Can you work these out from the model? Positions are in its coordinate system, mm. Coordinates: 2 decimals unless noted, no trailing zeros. Order: outer loops, then holes, each group sorted by start corner. A loop starts at its lowest first (then second) coordinate and runs counter-clockwise, first axis right, second up. Notation, with made-up numbers: (44, 1.5) - (69, 1.5) arc R27 ccw to (69, 22.5) - close; hole circle Ø3 at (-5, -29). An arc over 180 degrees is marked (long way). Return JSON: item names as keys, results as strings. Group by question number.
1) Imagine slicing it at C-C (y = -13.5). Write out the boundary of the cut face in (x, z), and give its area (3 significant figures).
2) If I drill on line 1 along Y through (x, z) = (436.5, 16.25); line 2 along Z through (x, y) = (182, -52); line 3 along Y through (x, z) = (67, 15.5), over which ranges is the centre line in solid material (lowest first)?
3) Imagine slicing it at B-B (z = 12). Give the number of separate pieces and of enclosed holes in the cut face, and give its area (3 significant figures).
4) For pin 1 Ø2 at (x, z) = (128.5, 10.5) entering from +Y; pin 2 Ø1 at (y, z) = (3, 17.5) entering from +X; pin 3 Ø1.5 at (x, z) = (218, 16) entering from +Y, each with a flat end and sliding along its axis, tell me the tip position at first contact or that it passes through.
5) Imagine slicing it at A-A (x = 46). Write out the boundary of the cut face in (y, z), and give its area (3 significant figures).
```python
from build123d import *

# Parameters (mm, degrees)
F0_W     = 505.468076095
F0_H     = 137.6467421651
F1_DEPTH = 7.366
F3_DEPTH = 12.446


# Not quite as in the source:
# - a feature names something its author has since deleted; it is built from what else it names


with BuildPart() as f1:
    # F0 (on Top) → F1 (new body)
    with BuildSketch(Plane.XY):
        with Locations((232.2135167196, 0.7967613637)):
            Rectangle(F0_W, F0_H)
    extrude(amount=F1_DEPTH)

    # F2 (on face) → F3 (join)
    with BuildSketch(Plane.XY.offset(7.366)):
        with BuildLine():
            Line((183.8642209768, 14.1799058765), (183.8642209768, 10.2725932375))
            Line((183.8642209768, 10.2725932375), (181.7528605461, 10.280970484))
            Line((181.7528605461, 10.280970484), (174.2617040873, 10.3483377025))
            Line((174.2617040873, 10.3483377025), (137.7773582935, 10.3483377025))
            Line((137.7773582935, 10.3483377025), (125.377446413, 4.0150946006))
            Line((125.377446413, 4.0150946006), (138.0158215761, -2.1848597098))
            Line((138.0158215761, -2.1848597098), (174.0232408047, -2.1848597098))
            Line((174.0232408047, -2.1848597098), (181.7289143801, -2.1529737648))
            Line((181.7289143801, -2.1529737648), (183.6102157831, -2.1509330043))
            Line((183.6102157831, -2.1509330043), (183.5907548666, -5.8423327282))
            Line((183.5907548666, -5.8423327282), (186.6615414619, -5.8423327282))
            Line((186.6615414619, -5.8423327282), (186.6615414619, -2.0806165412))
            Line((186.6615414619, -2.0806165412), (189.655572176, -2.0806165412))
            Line((189.655572176, -2.0806165412), (189.655572176, -5.8423327282))
            Line((189.655572176, -5.8423327282), (192.6495879889, -5.8423327282))
            Line((192.6495879889, -5.8423327282), (192.6495879889, -2.0806165412))
            Line((192.6495879889, -2.0806165412), (195.8739161491, -2.0806165412))
            Line((195.8739161491, -2.0806165412), (195.8739161491, -5.8423327282))
            Line((195.8739161491, -5.8423327282), (199.0982443094, -5.8423327282))
            Line((199.0982443094, -5.8423327282), (199.0982443094, -2.0806165412))
            Line((199.0982443094, -2.0806165412), (202.4761140347, -2.0806165412))
            Line((202.4761140347, -2.0806165412), (202.4761140347, -5.8423327282))
            Line((202.4761140347, -5.8423327282), (206.2378227711, -5.8423327282))
            Line((206.2378227711, -5.8423327282), (206.2378227711, -2.0806165412))
            Line((206.2378227711, -2.0806165412), (209.6156924963, -2.0806165412))
            Line((209.6156924963, -2.0806165412), (209.6156924963, -5.8423327282))
            Line((209.6156924963, -5.8423327282), (213.1471037865, -5.8423327282))
            Line((213.1471037865, -5.8423327282), (213.1471037865, -2.0806165412))
            Line((213.1471037865, -2.0806165412), (216.1411345005, -2.0806165412))
            Line((216.1411345005, -2.0806165412), (216.1411345005, -5.8423327282))
            Line((216.1411345005, -5.8423327282), (219.1351503134, -5.8423327282))
            Line((219.1351503134, -5.8423327282), (219.1351503134, -2.0806165412))
            Line((219.1351503134, -2.0806165412), (222.3594784737, -2.0806165412))
            Line((222.3594784737, -2.0806165412), (222.3594784737, -5.8423327282))
            Line((222.3594784737, -5.8423327282), (225.5838066339, -5.8423327282))
            Line((225.5838066339, -5.8423327282), (225.5838066339, -2.0806165412))
            Line((225.5838066339, -2.0806165412), (228.9616763592, -2.0806165412))
            Line((228.9616763592, -2.0806165412), (228.9616763592, -5.8423327282))
            Line((228.9616763592, -5.8423327282), (232.7233850956, -5.8423327282))
            Line((232.7233850956, -5.8423327282), (232.7233850956, -2.0806165412))
            Line((232.7233850956, -2.0806165412), (236.1012548208, -2.0806165412))
            Line((236.1012548208, -2.0806165412), (236.1012548208, -5.8423327282))
            Line((236.1012548208, -5.8423327282), (239.886666111, -5.8423327282))
            Line((239.886666111, -5.8423327282), (239.886666111, -2.0361929703))
            Line((239.886666111, -2.0361929703), (308.7113499641, -2.0361929703))
            Line((308.7113499641, -2.0361929703), (327.0893990993, -2.0361929703))
            ThreePointArc((327.0893990993, -2.0361929703), (338.0716042416, 0.4904142901), (346.8455672264, 7.5621996075))
            Line((346.8455672264, 7.5621996075), (379.0387098504, 16.6834991227))
            Line((379.0387098504, 16.6834991227), (375.7017479006, 19.6033408288))
            Line((375.7017479006, 19.6033408288), (379.0387098504, 23.4170116286))
            ThreePointArc((379.0387098504, 23.4170116286), (399.0077273508, 29.2230595274), (418.9767448512, 23.4170116286))
            Line((418.9767448512, 23.4170116286), (416.3737297058, 21.2878081948))
            Line((416.3737297058, 21.2878081948), (450.9352743626, 6.4515918493))
            Line((450.9352743626, 6.4515918493), (453.2975118055, 8.5896141827))
            Line((453.2975118055, 8.5896141827), (484.4302535057, 8.5896141827))
            Line((484.4302535057, 8.5896141827), (484.4302535057, 10.8214179054))
            Line((484.4302535057, 10.8214179054), (454.9943455488, 10.8214179054))
            Line((454.9943455488, 10.8214179054), (457.0494721473, 12.6347579062))
            Line((457.0494721473, 12.6347579062), (484.4302535057, 12.6347579062))
            Line((484.4302535057, 12.6347579062), (484.4302535057, 14.448097907))
            Line((484.4302535057, 14.448097907), (457.9519460917, 14.448097907))
            Line((457.9519460917, 14.448097907), (460.04427444, 16.5404137224))
            Line((460.04427444, 16.5404137224), (484.4302535057, 16.5404137224))
            Line((484.4302535057, 16.5404137224), (484.4302535057, 18.3537546545))
            Line((484.4302535057, 18.3537546545), (461.2901464378, 18.3537546545))
            Line((461.2901464378, 18.3537546545), (463.6734724045, 20.1696325094))
            Line((463.6734724045, 20.1696325094), (450.5897462368, 50.3342226148))
            Line((450.5897462368, 50.3342226148), (447.8478631112, 48.0109341443))
            ThreePointArc((447.8478631112, 48.0109341443), (399.0077273508, 55.560682533), (350.1675915904, 48.0109341443))
            Line((350.1675915904, 48.0109341443), (348.1977880001, 45.759730041))
            Line((348.1977880001, 45.759730041), (345.6249833107, 48.0109341443))
            Line((345.6249833107, 48.0109341443), (336.9521223247, 17.9653423708))
            ThreePointArc((336.9521223247, 17.9653423708), (327.6334286446, 12.1000348485), (316.7435458205, 10.4720494957))
            Line((316.7435458205, 10.4720494957), (309.5143437386, 10.3298625909))
            Line((309.5143437386, 10.3298625909), (239.8866713047, 10.3298625909))
            Line((239.8866713047, 10.3298625909), (239.8866713047, 14.1799058765))
            Line((239.8866713047, 14.1799058765), (236.3552600145, 14.1799058765))
            Line((236.3552600145, 14.1799058765), (236.3552600145, 10.4181896895))
            Line((236.3552600145, 10.4181896895), (232.9773902893, 10.4181896895))
            Line((232.9773902893, 10.4181896895), (232.9773902893, 14.1799058765))
            Line((232.9773902893, 14.1799058765), (229.2156815529, 14.1799058765))
            Line((229.2156815529, 14.1799058765), (229.2156815529, 10.4181896895))
            Line((229.2156815529, 10.4181896895), (225.8378118277, 10.4181896895))
            Line((225.8378118277, 10.4181896895), (225.8378118277, 14.1799058765))
            Line((225.8378118277, 14.1799058765), (222.6134836674, 14.1799058765))
            Line((222.6134836674, 14.1799058765), (222.6134836674, 10.4181896895))
            Line((222.6134836674, 10.4181896895), (219.3891555071, 10.4181896895))
            Line((219.3891555071, 10.4181896895), (219.3891555071, 14.1799058765))
            Line((219.3891555071, 14.1799058765), (216.3951396942, 14.1799058765))
            Line((216.3951396942, 14.1799058765), (216.3951396942, 10.4181896895))
            Line((216.3951396942, 10.4181896895), (213.4011089802, 10.4181896895))
            Line((213.4011089802, 10.4181896895), (213.4011089802, 14.1799058765))
            Line((213.4011089802, 14.1799058765), (209.86969769, 14.1799058765))
            Line((209.86969769, 14.1799058765), (209.86969769, 10.4181896895))
            Line((209.86969769, 10.4181896895), (206.4918279648, 10.4181896895))
            Line((206.4918279648, 10.4181896895), (206.4918279648, 14.1799058765))
            Line((206.4918279648, 14.1799058765), (202.7301192284, 14.1799058765))
            Line((202.7301192284, 14.1799058765), (202.7301192284, 10.4181896895))
            Line((202.7301192284, 10.4181896895), (199.3522495031, 10.4181896895))
            Line((199.3522495031, 10.4181896895), (199.3522495031, 14.1799058765))
            Line((199.3522495031, 14.1799058765), (196.1279213428, 14.1799058765))
            Line((196.1279213428, 14.1799058765), (196.1279213428, 10.4181896895))
            Line((196.1279213428, 10.4181896895), (192.9035931826, 10.4181896895))
            Line((192.9035931826, 10.4181896895), (192.9035931826, 14.1799058765))
            Line((192.9035931826, 14.1799058765), (189.9095773697, 14.1799058765))
            Line((189.9095773697, 14.1799058765), (189.9095773697, 10.4181896895))
            Line((189.9095773697, 10.4181896895), (186.9155466557, 10.4181896895))
            Line((186.9155466557, 10.4181896895), (186.9155466557, 14.1799058765))
            Line((186.9155466557, 14.1799058765), (183.8642209768, 14.1799058765))
        make_face()
        with BuildLine():
            Line((370.6372472565, 23.5322912479), (374.053896924, 27.4370337251))
            ThreePointArc((374.053896924, 27.4370337251), (399.0077273508, 33.7810246324), (423.9615577776, 27.4370337251))
            Line((423.9615577776, 27.4370337251), (421.708929064, 25.8076728149))
            ThreePointArc((421.708929064, 25.8076728149), (399.0077273508, 31.9265013842), (376.3065256376, 25.8076728149))
            Line((376.3065256376, 25.8076728149), (372.7205432622, 21.7094072429))
            Line((372.7205432622, 21.7094072429), (370.6372472565, 23.5322912479))
        make_face(mode=Mode.SUBTRACT)
        with BuildLine():
            Line((365.6382056992, 28.3170708711), (368.6322219076, 31.7388036808))
            ThreePointArc((368.6322219076, 31.7388036808), (399.0077273508, 38.526410097), (429.383232794, 31.7388036808))
            Line((429.383232794, 31.7388036808), (426.7392740049, 29.867535424))
            ThreePointArc((426.7392740049, 29.867535424), (399.0077273508, 36.4081558373), (371.2761806967, 29.867535424))
            Line((371.2761806967, 29.867535424), (368.0630232644, 26.1953555015))
            Line((368.0630232644, 26.1953555015), (365.6382056992, 28.3170708711))
        make_face(mode=Mode.SUBTRACT)
        with BuildLine():
            Line((360.4813304683, 33.5443242144), (363.4392711441, 36.9248278439))
            ThreePointArc((363.4392711441, 36.9248278439), (399.0077273508, 44.2750490819), (434.5761835575, 36.9248278439))
            Line((434.5761835575, 36.9248278439), (432.3772490025, 35.0923612714))
            ThreePointArc((432.3772490025, 35.0923612714), (399.0077273508, 42.2705737087), (365.6382056992, 35.0923612714))
            Line((365.6382056992, 35.0923612714), (362.6348697567, 31.6599773371))
            Line((362.6348697567, 31.6599773371), (360.4813304683, 33.5443242144))
        make_face(mode=Mode.SUBTRACT)
        with BuildLine():
            Line((355.3299033536, 38.152305195), (358.0891265806, 41.3057031687))
            ThreePointArc((358.0891265806, 41.3057031687), (399.0077273508, 48.9346794019), (439.926328121, 41.3057031687))
            Line((439.926328121, 41.3057031687), (436.997769417, 39.1854137116))
            ThreePointArc((436.997769417, 39.1854137116), (399.0077273508, 46.6356083993), (361.0176852847, 39.1854137116))
            Line((361.0176852847, 39.1854137116), (358.0393189878, 35.7815665152))
            Line((358.0393189878, 35.7815665152), (355.3299033536, 38.152305195))
        make_face(mode=Mode.SUBTRACT)
        with BuildLine():
            Line((350.1675915904, 43.2099050709), (352.5468626356, 45.9290719797))
            ThreePointArc((352.5468626356, 45.9290719797), (399.0077273508, 53.6790820799), (445.468592066, 45.9290719797))
            Line((445.468592066, 45.9290719797), (442.4422114296, 43.5071010637))
            ThreePointArc((442.4422114296, 43.5071010637), (399.0077273508, 51.1039718638), (355.573243272, 43.5071010637))
            Line((355.573243272, 43.5071010637), (353.0819166526, 40.6598706415))
            Line((353.0819166526, 40.6598706415), (350.1675915904, 43.2099050709))
        make_face(mode=Mode.SUBTRACT)
        Polygon((108.4468066692, -2.1848597098), (122.0492497087, 3.6468699109), (108.5446923971, 10.3483377025), (-20.3237645328, 10.3483377025), (-20.5205213279, -2.1848597098), align=None)
    extrude(amount=F3_DEPTH)


solid = f1.part
```
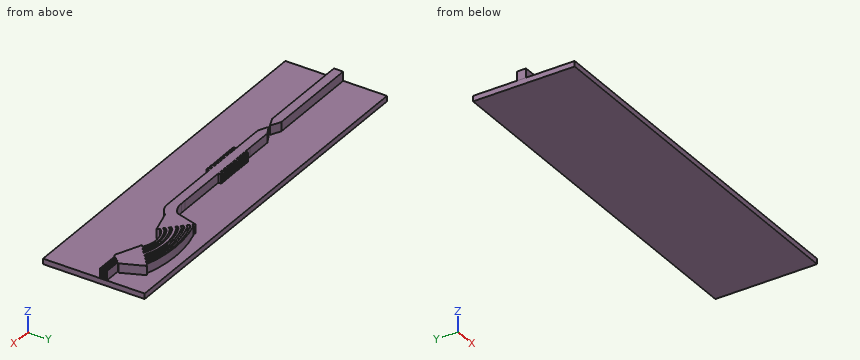
Calculated:
{
 "1": {"outline": "(-20.52, 0) - (484.95, 0) - (484.95, 7.37) - (-20.52, 7.37) - close", "area": "3,720 mm2"},
 "2": {"line 1": "12.65 to 39.39, 42.57 to 45.49, 48.68 to 51.16", "line 2": "0 to 7.37", "line 3": "-2.18 to 10.35"},
 "3": {"separate pieces": "2", "enclosed holes": "5", "area": "7,910 mm2"},
 "4": {"pin 1": "y = 6.12", "pin 2": "x = 342.83", "pin 3": "y = 14.18"},
 "5": {"outline": "(-68.03, 0) - (69.62, 0) - (69.62, 7.37) - (10.35, 7.37) - (10.35, 19.81) - (-2.18, 19.81) - (-2.18, 7.37) - (-68.03, 7.37) - close", "area": "1,170 mm2"}
}
